For this review, take the finished solid that the model builds, in its own axes (mm). A direction names the side the tool comes from. Coordinates: 2 decimals unless noted, no trailing zeros. Order: outer loops, then holes, each group sorted by start corner. A loop starts at its lowest first (then second) coordinate and runs counter-clockwise, first axis right, second up. Notation, with made-up numbers: (38.25, 62.25) -> (57.25, 62.25) arc R35 cw to (57.25, 100.25) -> close; hole circle Ø7 at (-32.75, 30). An arc over 180 degrees is marked (long way). Write item = value, one per line. Start each with the question number.
1) Insertion check: pin 1 Ø14.5 at (x, z) = (-1.5, 0) entering from -Y (3 decimals); pin 2 Ø3 at (y, z) = (-4.5, -63.5) entering from +X; pin 3 Ø4 at (y, z) = (-8, -67) entering from -X. Each pin has a flat end and moves straight along its axis. Give the tip position at first contact, or say it passes through.
2) Consider section A-A on y = 4. Give the boundary of the cut face in (x, z) (1 decimal).
3) Consider section D-D on z = 1. Give the boundary of the cut face in (x, y) (1 decimal), and give its area (3 significant figures).
4) Consider section B-B on x = -30. Give the boundary of the cut face in (y, z) (1 decimal).
5) Draft analysis for pull direction Z (two halves, no side actions). For faces 4 (the face through (-16, 15.24, -34)), 5 (the face through (-3.298, -0.133, 0.123)), state which applies: +Z half, -Z half, draft (parallel to the pull), parting line (faces both ways), or undercut.
6) Machinability: for faces 1 (the face through (-45.974, -7, 0)), 2 (the face through (17.272, 11, 6)), 3 (the face through (-38.347, -0.133, -68.83)), which of the approach directions +Z, -Z, +X, -X, +Y, -Y give a long, thin tool a straight path to every point of the face, cutting with its end or side? Answer none if there is none.
7) Wall thickness on probe 1 along Z at (x, y) = (-9.5, 9) (1 decimal); probe 2 along X at (y, z) = (11, -25); probe 3 along Z at (x, y) = (-37, 12.5): over which ranges is each line inside the solid? List them lowest first. Write a range as [from, to].
8) Consider section C-C on y = -11. Give the boundary of the cut face in (x, z), and give its area (3 significant figures).
from build123d import *

# Parameters (mm, degrees)
F0_W      = 6.35
F0_H      = 28.575
F1_DEPTH  = 9.525
F2_DEPTH  = 12.7
F3_DEPTH  = 15.24
F4_DEPTH  = 12.7
F5_W      = 6.35
F5_H      = 28.575
F6_DEPTH  = 4.826
F7_DEPTH  = 12.7
F8_DEPTH  = 15.24
F9_DEPTH  = 12.7
F10_W     = 6.35
F10_H     = 28.575
F11_DEPTH = 4.826


with BuildPart() as f1:
    # F0 (on Front) → F1 (new body, symmetric)
    with BuildSketch(Plane.XZ):
        with Locations((-49.149, 0)):
            Rectangle(F0_W, F0_H)
        Polygon((17.272, 14.2875), (-45.974, 14.2875), (-45.974, -14.2875), (21.082, -14.2875), (23.749, -14.2875), (34.798, -3.2385), (17.272, -3.2385), align=None)
        with BuildLine():
            Line((-32.760566, 5.588), (-8.884566, 5.588))
            ThreePointArc((-8.884566, 5.588), (-3.296566, 0), (-8.884566, -5.588))
            Line((-8.884566, -5.588), (-32.760566, -5.588))
            ThreePointArc((-32.760566, -5.588), (-38.348566, 0), (-32.760566, 5.588))
        make_face(mode=Mode.SUBTRACT)
        Polygon((-45.974, -14.2875), (-52.324, -14.2875), (-52.324, -34.3535), (21.082, -34.3535), (21.082, -14.2875), align=None)
        Polygon((52.324, 14.2875), (17.272, 14.2875), (17.272, -3.2385), (34.798, -3.2385), align=None)
        Polygon((21.082, -34.3535), (-52.324, -34.3535), (-52.324, -54.4195), (-45.974, -54.4195), (21.082, -54.4195), align=None)
        Polygon((52.324, -14.2875), (52.324, 14.2875), (34.798, -3.2385), (23.749, -14.2875), align=None)
        with Locations((-49.149, -68.707)):
            Rectangle(F0_W, F0_H)
        Polygon((23.749, -54.4195), (21.082, -54.4195), (-45.974, -54.4195), (-45.974, -82.9945), (17.272, -82.9945), (17.272, -65.4685), (34.798, -65.4685), align=None)
        with BuildLine():
            ThreePointArc((-8.884566, -63.119), (-3.296566, -68.707), (-8.884566, -74.295))
            Line((-8.884566, -74.295), (-32.760566, -74.295))
            ThreePointArc((-32.760566, -74.295), (-38.348566, -68.707), (-32.760566, -63.119))
            Line((-32.760566, -63.119), (-8.884566, -63.119))
        make_face(mode=Mode.SUBTRACT)
        Polygon((52.324, -54.4195), (23.749, -54.4195), (34.798, -65.4685), (52.324, -82.9945), align=None)
        Polygon((52.324, -82.9945), (34.798, -65.4685), (17.272, -65.4685), (17.272, -82.9945), align=None)
    extrude(amount=F1_DEPTH, both=True)

    # F0 (on Front) → F2 (cut, symmetric)
    with BuildSketch(Plane.XZ):
        Polygon((52.324, -14.2875), (52.324, 14.2875), (34.798, -3.2385), (23.749, -14.2875), align=None)
    extrude(amount=F2_DEPTH, both=True, mode=Mode.SUBTRACT)

    # F0 (on Front) → F3 (join, symmetric)
    with BuildSketch(Plane.XZ):
        Polygon((-45.974, -14.2875), (-52.324, -14.2875), (-52.324, -34.3535), (21.082, -34.3535), (21.082, -14.2875), align=None)
    extrude(amount=F3_DEPTH, both=True)

    # F0 (on Front) → F4 (join, symmetric)
    with BuildSketch(Plane.XZ):
        Polygon((52.324, 14.2875), (17.272, 14.2875), (17.272, -3.2385), (34.798, -3.2385), align=None)
    extrude(amount=F4_DEPTH, both=True)

    # F5 (on face) → F6 (cut)
    with BuildSketch(Plane.XZ.offset(9.525)):
        with Locations((-49.149, 0)):
            Rectangle(F5_W, F5_H)
    extrude(amount=-F6_DEPTH, mode=Mode.SUBTRACT)

    # F0 (on Front) → F7 (cut, symmetric)
    with BuildSketch(Plane.XZ):
        Polygon((52.324, -54.4195), (23.749, -54.4195), (34.798, -65.4685), (52.324, -82.9945), align=None)
    extrude(amount=F7_DEPTH, both=True, mode=Mode.SUBTRACT)

    # F0 (on Front) → F8 (join, symmetric)
    with BuildSketch(Plane.XZ):
        Polygon((21.082, -34.3535), (-52.324, -34.3535), (-52.324, -54.4195), (-45.974, -54.4195), (21.082, -54.4195), align=None)
    extrude(amount=F8_DEPTH, both=True)

    # F0 (on Front) → F9 (join, symmetric)
    with BuildSketch(Plane.XZ):
        Polygon((52.324, -82.9945), (34.798, -65.4685), (17.272, -65.4685), (17.272, -82.9945), align=None)
    extrude(amount=F9_DEPTH, both=True)

    # F10 (on face) → F11 (cut)
    with BuildSketch(Plane.XZ.offset(9.525)):
        with Locations((-49.149, -68.707)):
            Rectangle(F10_W, F10_H)
    extrude(amount=-F11_DEPTH, mode=Mode.SUBTRACT)


solid = f1.part
Answer sheet:
q1.pin_1 = -9.525
q1.pin_2 = 34.33
q1.pin_3 = -45.97
q2.outline = (-52.3, -83) -> (52.3, -83) -> (23.7, -54.4) -> (21.1, -54.4) -> (21.1, -14.3) -> (23.7, -14.3) -> (52.3, 14.3) -> (-52.3, 14.3) -> close; hole (-32.8, -74.3) -> (-8.9, -74.3) arc R5.6 ccw to (-8.9, -63.1) -> (-32.8, -63.1) arc R5.6 ccw to start; hole (-32.8, -5.6) -> (-8.9, -5.6) arc R5.6 ccw to (-8.9, 5.6) -> (-32.8, 5.6) arc R5.6 ccw to start
q3.outline = (-52.3, -4.7) -> (-46, -4.7) -> (-46, -9.5) -> (-38.3, -9.5) -> (-38.3, 9.5) -> (-52.3, 9.5) -> close; (-3.4, -9.5) -> (17.3, -9.5) -> (17.3, -12.7) -> (39, -12.7) -> (39, 12.7) -> (17.3, 12.7) -> (17.3, 9.5) -> (-3.4, 9.5) -> close
q3.area = 1,180 mm2
q4.outline = (-15.2, -54.4) -> (-9.5, -54.4) -> (-9.5, -63.1) -> (9.5, -63.1) -> (9.5, -54.4) -> (15.2, -54.4) -> (15.2, -14.3) -> (9.5, -14.3) -> (9.5, -5.6) -> (-9.5, -5.6) -> (-9.5, -14.3) -> (-15.2, -14.3) -> close; (-9.5, -83) -> (9.5, -83) -> (9.5, -74.3) -> (-9.5, -74.3) -> close; (-9.5, 5.6) -> (9.5, 5.6) -> (9.5, 14.3) -> (-9.5, 14.3) -> close
q5.face_4 = draft
q5.face_5 = undercut
q6.face_1 = +Z, -X, -Y
q6.face_2 = +Z, -X, +Y
q6.face_3 = +Y, -Y
q7.probe_1 = [-83, -74.3], [-63.1, -5.6], [5.6, 14.3]
q7.probe_2 = [-52.32, 21.08]
q7.probe_3 = [-54.42, -14.29]
q8.outline = (-52.32, -54.42) -> (21.08, -54.42) -> (21.08, -14.29) -> (-52.32, -14.29) -> close; (17.27, -82.99) -> (52.32, -82.99) -> (34.8, -65.47) -> (17.27, -65.47) -> close; (17.27, -3.24) -> (34.8, -3.24) -> (52.32, 14.29) -> (17.27, 14.29) -> close
q8.area = 3,870 mm2
